```python
from build123d import *

# Parameters (mm, degrees)
F1_DEPTH = 101.6
F2_W     = 101.6
F2_H     = 76.2
F3_DEPTH = 127.001


with BuildPart() as f1:
    # F0 (on Front) → F1 (new body, symmetric)
    with BuildSketch(Plane.XZ):
        with BuildLine():
            Line((0, 50.8), (0, 0))
            Line((0, 0), (127, 0))
            Line((127, 0), (127, 152.4))
            Line((127, 152.4), (101.6, 152.4))
            ThreePointArc((101.6, 152.4), (63.692052, 88.707948), (0, 50.8))
        make_face()
    extrude(amount=F1_DEPTH, both=True)

    # F2 (on face) → F3 (cut, through all)
    with BuildSketch(Plane.YZ.offset(127)):
        with Locations((0, 114.3)):
            Rectangle(F2_W, F2_H)
    extrude(amount=-F3_DEPTH, mode=Mode.SUBTRACT)


solid = f1.part
```
Geometry: final body of the model. Coordinates: model frame, mm. A direction names the side the tool comes from. Give positions to 0.01 mm unless a question says otherwise; leave off trailing zeros. Loops run counter-clockwise (first coordinate to the right, second up) from the corner with the lowest first, then second, coordinate; pieces in that order, holes last. Notation, with made-up numbers: (-10.5, 9) - (31.5, 9) arc R9 ccw to (31.5, 21) - close; hole circle Ø7 at (-34.5, 84.5). An arc over 180 degrees is marked (long way). Answer as CSV lines item,"result". Start each with the question number.
(1) Section query C-C (y = -38.5). Output: boundary loops of the cut face in (x, z), and give its area (3 significant figures).
(2) Ray query, line 1 along Y through (x, z) = (112, 107.5); line 2 along Z through (x, y) = (8, -66.5); line 3 along Z through (x, y) = (85, 47). Return the intervals inside material, ascending. Write a range as [from, to].
(3) Section query B-B (z = 124.5). Output: boundary loops of the cut face in (x, y), and give its area (3 significant figures).
(4) Reachability of faces 5 (the face through (89, -1, 76.2)), 6 (the face through (38.643, -1.422, 68.517)) from +Z, -Z, +X, -X, +Y, -Y: full face, straight path, thin tool, end or side. Return the list, or none.
(5) Pin query (flat end, axial travel): P1, Ø8, axis at x = 18, y = -35.5, coming from the +Z side; P2, Ø23, axis at x = 100.5, y = -21, coming from the +Z side; P3, Ø12, axis at x = 89.5, y = 78.5, coming from the +Z side. Return the tip coordinate at first contact, or that it passes through.
(6) Section query D-D (z = 80). Output: boundary loops of the cut face in (x, y), and give its area (3 significant figures).
(7) Mould query, pull axis Y, two halves, no side actions, for faces 1 (the face through (97, 50.8, 105)), 2 (the face through (97, -50.8, 105)), 3 (the face through (77, 101.6, 60)), 4 (the face through (63, -1, 0)). Classes: +Y half, -Y half, draft (parallel to the pull), parting line (faces both ways), or undercut.
(8) Section query A-A (x = 118.5). Output: boundary loops of the cut face in (y, z), and give its area (3 significant figures).
Worked answers:
1,outline,"(0, 0) - (127, 0) - (127, 76.2) - (49.51, 76.2) arc R150.66 cw to (0, 50.8) - close"
1,area,"8,950 mm^2"
2,line 1,"y = [-101.6, -50.8], [50.8, 101.6]"
2,line 2,"z = [0, 53.42]"
2,line 3,"z = [0, 76.2]"
3,outline,"(90.18, -101.6) - (127, -101.6) - (127, -50.8) - (90.18, -50.8) - close; (90.18, 50.8) - (127, 50.8) - (127, 101.6) - (90.18, 101.6) - close"
3,area,"3,740 mm^2"
4,face 5,"+Z, +X, -X"
4,face 6,"+Z, -X, +Y, -Y"
5,P1,"stops at z = 59.25"
5,P2,"stops at z = 76.2"
5,P3,"stops at z = 135.57"
6,outline,"(54.21, -101.6) - (127, -101.6) - (127, -50.8) - (54.21, -50.8) - close; (54.21, 50.8) - (127, 50.8) - (127, 101.6) - (54.21, 101.6) - close"
6,area,"7,400 mm^2"
7,face 1,"undercut"
7,face 2,"undercut"
7,face 3,"+Y half"
7,face 4,"draft"
8,outline,"(-101.6, 0) - (101.6, 0) - (101.6, 152.4) - (50.8, 152.4) - (50.8, 76.2) - (-50.8, 76.2) - (-50.8, 152.4) - (-101.6, 152.4) - close"
8,area,"23,200 mm^2"
